Geometry check sheet. Reference: drawing and pictorial views, mm from the part's lowest x, y, z. Give positions to 0.01 mm unless a question says otherwise; leave off trailing zeros. Loops run counter-clockwise (first coordinate to the right, second up) from the corner with the lowest first, then second, coordinate; pieces in that order, holes last. Notation, with made-up numbers: (-7, 43) -> (21, 43) arc R13 cw to (21, 52) -> close; hole circle Ø5 at (-35.5, 78.25). An arc over 180 degrees is marked (long way). Answer in a Markdown table with one row per item. Add a question column.
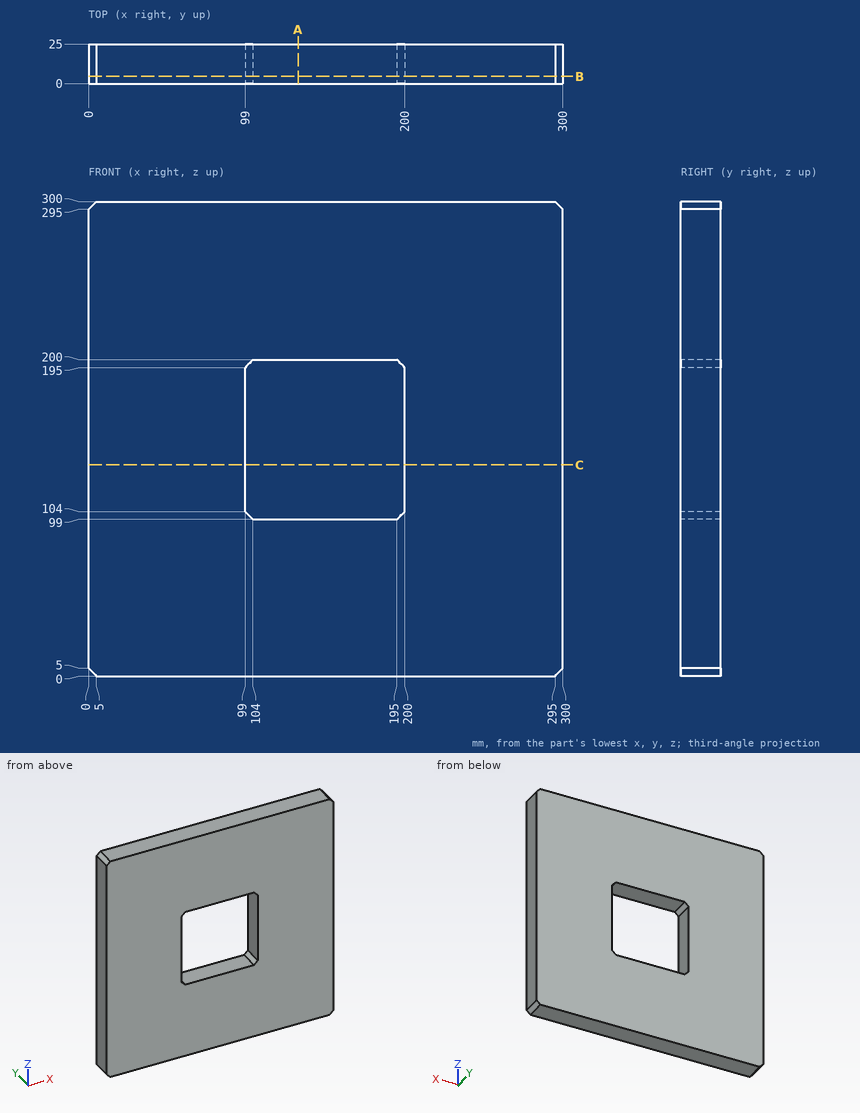
1. Sectioned sample at A-A (x = 132.5). Enter the section's corners in (y, z).
2. Sectioned sample at B-B (y = 4.5). Enter the section's corners in (x, z), plus the area to 3 significant figures.
3. Material ranges on L1, parallel to Z at x = 154, y = 2, recorded low to high. Write a range as from..to.
4. Sectioned sample at C-C (z = 133.5). Enter the section's corners in (x, y), plus the area to 4 significant figures.
Response:
| question | item | result |
|---|---|---|
| 1 | outline | (0, 0) -> (25, 0) -> (25, 99) -> (0, 99) -> close; (0, 200) -> (25, 200) -> (25, 300) -> (0, 300) -> close |
| 2 | outline | (0, 5) -> (5, 0) -> (295, 0) -> (300, 5) -> (300, 295) -> (295, 300) -> (5, 300) -> (0, 295) -> close; hole (99, 104) -> (104, 99) -> (195, 99) -> (200, 104) -> (200, 195) -> (195, 200) -> (104, 200) -> (99, 195) -> close |
| 2 | area | 79,800 mm2 |
| 3 | L1 | z = 0..99, 200..300 |
| 4 | outline | (0, 0) -> (99, 0) -> (99, 25) -> (0, 25) -> close; (200, 0) -> (300, 0) -> (300, 25) -> (200, 25) -> close |
| 4 | area | 4,975 mm2 |
